```python
from build123d import *

# Parameters (mm, degrees)
SKETCH1_R           = 2.38125
BOSS_EXTRUDE1_DEPTH = 3.175
CAVITY1_START       = -3.175
CAVITY1_OUTLINE_W   = 1.236627981
CAVITY1_OUTLINE_H   = 3.175
CAVITY1_DEPTH       = 3.175
CAVITY1_START_2     = 12.7
CAVITY1_2_OUTLINE_W = 1.236627981
CAVITY1_2_OUTLINE_H = 3.175
CAVITY1_2_DEPTH     = 3.175


# Read off the part's stored shape, not the designer's step: Cavity1
with BuildPart() as part:
    # Sketch1 → Boss-Extrude1 (new body)
    with BuildSketch(Plane.XY):
        with BuildLine():
            Line((0, -1.722993842), (12.7, -1.722993842))
            Line((12.7, -1.722993842), (12.7, 3.175))
            Line((12.7, 3.175), (15.875, 3.175))
            Line((15.875, 3.175), (15.875, 12.264476338))
            ThreePointArc((15.875, 12.264476338), (14.015128061, 16.754604399), (9.525, 18.614476338))
            Line((9.525, 18.614476338), (3.175, 18.614476338))
            ThreePointArc((3.175, 18.614476338), (-1.315128061, 16.754604399), (-3.175, 12.264476338))
            Line((-3.175, 12.264476338), (-3.175, 3.175))
            Line((-3.175, 3.175), (0, 3.175))
            Line((0, 3.175), (0, -1.722993842))
        make_face()
        with Locations((6.35, 8.437006158)):
            Circle(SKETCH1_R, mode=Mode.SUBTRACT)
    extrude(amount=BOSS_EXTRUDE1_DEPTH)

    # Cavity1 outline → Cavity1 (cut)
    with BuildSketch(Plane.YZ.offset(CAVITY1_START)):
        with Locations((3.793313991, 1.5875)):
            Rectangle(CAVITY1_OUTLINE_W, CAVITY1_OUTLINE_H)
    extrude(amount=CAVITY1_DEPTH, mode=Mode.SUBTRACT)

    # Cavity1 2 outline → Cavity1 2 (cut)
    with BuildSketch(Plane.YZ.offset(CAVITY1_START_2)):
        with Locations((3.793313991, 1.5875)):
            Rectangle(CAVITY1_2_OUTLINE_W, CAVITY1_2_OUTLINE_H)
    extrude(amount=CAVITY1_2_DEPTH, mode=Mode.SUBTRACT)


solid = part.part
```
Source: CAD feature listing. Evaluate the final solid. Frame: model axes, mm. A direction names the side the tool comes from. Give positions to 0.01 mm unless a question says otherwise; leave off trailing zeros. Loops run counter-clockwise (first coordinate to the right, second up) from the corner with the lowest first, then second, coordinate; pieces in that order, holes last. Notation, with made-up numbers: (88.25, 1) -> (124.25, 1) arc R30 ccw to (124.25, 23) -> close; hole circle Ø8 at (-4, 46.25). An arc over 180 degrees is marked (long way). Use a Markdown table: item, result. Add a question column.
(1) Ray query, line 1 (Y direction, x = 6.35, z = 2.1); line 2 (Y direction, x = 8.5, z = 1.65); line 3 (X direction, y = 2.75, z = 1.4). Return the intervals inside material, ascending.
(2) Section query A-A (x = 6.35). Output: boundary loops of the cut face in (y, z) (3 decimals).
(3) Pull-direction query (Y, two-part tool) for faces 1 (the face through (-1.27, 16.8, 1.57)), 2 (the face through (-3.175, 8, 2)), 3 (the face through (4.595, 10.046, 1.565)); classes: +Y half, -Y half, draft (parallel to the pull), parting line (faces both ways), or undercut.
(4) Access query for faces 4 (the face through (-2, 4.412, 2)), 5 (the face through (15.875, 8, 2)), 6 (the face through (14, 4.412, 2)). Directions: +Z, -Z, +X, -X, +Y, -Y. A direction counts if a zero-diameter tool reaches every point of the face in a straight line with its end or side. Return the directions, or none.
(5) First-contact query: pin 1 Ø1.5 at (y, z) = (1, 2.5) entering from -X. Flat tip, straight axial feed; report the tip coordinate or a pass-through.
(6) Section query D-D (y = 2). Output: boundary loops of the cut face in (x, z) (3 decimals).
(7) Section query B-B (y = 7.5). Output: boundary loops of the cut face in (x, z) (3 decimals), then the cut area to 3 significant figures.
Checked values:
| question | item | result |
|---|---|---|
| 1 | line 1 | -1.72 to 6.06, 10.82 to 18.61 |
| 1 | line 2 | -1.72 to 7.41, 9.46 to 18.61 |
| 1 | line 3 | 0 to 12.7 |
| 2 | outline | (-1.723, 0) -> (6.056, 0) -> (6.056, 3.175) -> (-1.723, 3.175) -> close; (10.818, 0) -> (18.614, 0) -> (18.614, 3.175) -> (10.818, 3.175) -> close |
| 3 | face 1 | +Y half |
| 3 | face 2 | draft |
| 3 | face 3 | undercut |
| 4 | face 4 | +Z, -Z, -X, -Y |
| 4 | face 5 | +Z, -Z, +X, +Y, -Y |
| 4 | face 6 | +Z, -Z, +X, -Y |
| 5 | pin 1 | x = 0 |
| 6 | outline | (0, 0) -> (12.7, 0) -> (12.7, 3.175) -> (0, 3.175) -> close |
| 7 | outline | (-3.175, 0) -> (4.161, 0) -> (4.161, 3.175) -> (-3.175, 3.175) -> close; (8.539, 0) -> (15.875, 0) -> (15.875, 3.175) -> (8.539, 3.175) -> close |
| 7 | area | 46.6 mm^2 |
